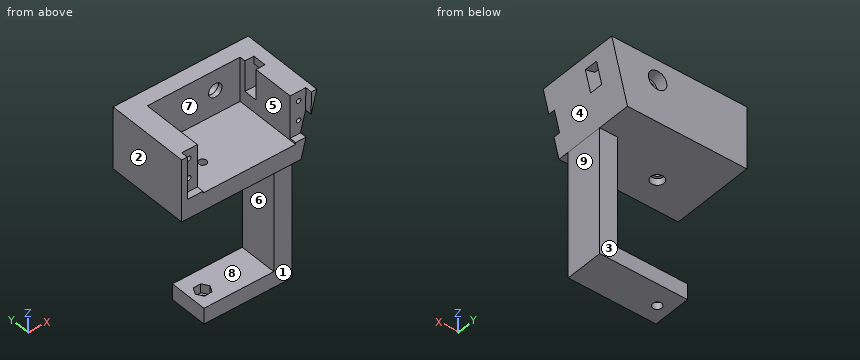
Autodesk Inventor part; units mm, degrees
ref_plane "Work Plane4" through (-33.8514, -22.438, 35.052) normal (0, 0, 1) x (0, 1, 0)
ref_plane "YZ Plane" through (0, 0, 0) normal (1, 0, 0) x (0, 1, 0)
ref_plane "XZ Plane" through (0, 0, 0) normal (0, 1, 0) x (-1, 0, 0)
sketch "Sketch1" plane through (0, 0, 0) normal (0, 0, 1) x (1, 0, 0)
  line L0 (-33.8514, 24.552) -> (33.4586, 24.552)
  line L1 (33.4586, 24.552) -> (33.4586, -22.438)
  line L2 (33.4586, -22.438) -> (-33.8514, -22.438)
  line L3 (-33.8514, -22.438) -> (-33.8514, 24.552)
  line L4 (33.4586, -22.438) -> (33.4586, -16.088)
  line L5 (33.4586, -16.088) -> (23.2986, -16.088)
  line L6 (23.2986, -16.088) -> (23.2986, 5.502)
  line L7 (23.2986, 5.502) -> (33.4586, 5.502)
  point P0 (0, 0)
  dimension "d0" = 67.31
  dimension "d1" = 46.99
  dimension "d10" = 6.35
  dimension "d11" = 10.16
  dimension "d12" = 21.59
ref_plane "Work Plane3" through (-33.8514, -22.438, 0) normal (0, 0, 1) x (0, 1, 0)
ref_plane "Work Plane4" through (-33.8514, -22.438, 35.052) normal (0, 0, 1) x (0, 1, 0)
sketch "Sketch3" plane through (-33.8514, -22.438, 35.052) normal (0, 0, 1) x (0, 1, 0)
  line L0 (0, 0) -> (46.99, 0)
  line L1 (46.99, 0) -> (46.99, -76.2)
  line L2 (46.99, -76.2) -> (0, -76.2)
  line L3 (0, -76.2) -> (0, 0)
  point P0 (22.438, -33.8514)
  dimension "d4" = 46.99
  dimension "d5" = 76.2
loft "Loft1" add profiles "Sketch3", "Sketch1"
sketch "Sketch5" plane through (33.4586, -22.438, 0) normal (0, 0, -1) x (-1, 0, 0)
  line L0 (67.31, 0) -> (67.31, 46.99)
  line L1 (-8.89, 0) -> (67.31, 0)
  circle A0 centre (42.037, 16.383) radius 3.683
  circle A1 centre (42.037, 16.383) radius 2.159
  point P0 (33.4586, 22.438)
  dimension "d17" = 7.366
  dimension "d20" = 4.318
extrude "Extrusion1" add sketch "Sketch1" against normal blind 71.12 contours L1 L5 L6 L7
extrude "Extrusion4" cut sketch "Sketch5" along normal through all both and the other way through all contours A1
extrude "Extrusion5" cut sketch "Sketch5" against normal blind 3.81 contours A0 | A1
sketch "Sketch7" plane through (23.2986, -16.088, 0) normal (-1, 0, 0) x (0, 0, 1)
  point P0 (0, 16.088)
sketch "Sketch8" plane through (23.2986, -16.088, 0) normal (-1, 0, 0) x (0, 0, 1)
  line L0 (0, 0) -> (-71.12, 0)
  line L1 (0, 21.59) -> (-71.12, 21.59)
  line L2 (-71.12, 0) -> (-62.23, 0)
  line L3 (-62.23, 0) -> (-62.23, 21.59)
  line L4 (-62.23, 21.59) -> (-71.12, 21.59)
  line L5 (-71.12, 21.59) -> (-71.12, 0)
  point P0 (0, 16.088)
  dimension "d27" = 8.89
extrude "Extrusion6" add sketch "Sketch8" along normal blind 39.37
sketch "Sketch9" plane through (0, 0, -71.12) normal (0, 0, -1) x (-1, 0, 0)
  line L0 (16.0714, 5.502) -> (16.0714, -16.088)
  line L1 (-33.4586, -16.088) -> (16.0714, -16.088)
  circle A0 centre (8.5784, -6.055) radius 2.54
  point P0 (0, 0)
  dimension "d34" = 5.08
extrude "Extrusion7" cut sketch "Sketch9" against normal blind 39.37
sketch "Sketch10" plane through (-33.8514, -22.438, 35.052) normal (0, -1, 0) x (1, 0, 0)
  line L0 (67.31, -35.052) -> (67.31, -106.172)
  line L1 (67.31, -35.052) -> (70.1199, -23.9728)
  line L2 (76.2, 0) -> (67.31, -35.052)
  line L3 (70.1199, -23.9728) -> (64.2779, -23.9728)
  line L4 (64.2779, -23.9728) -> (64.2779, -24.9888)
  line L5 (64.2779, -24.9888) -> (11.9539, -24.9888)
  line L6 (11.9539, -24.9888) -> (11.9539, -23.9728)
  line L7 (11.9539, -23.9728) -> (3.1655, -23.9728)
  line L8 (3.1655, -23.9728) -> (3.1655, 0)
  line L9 (0, 0) -> (76.2, 0)
  line L10 (76.2, 0) -> (73.0154, -12.5564)
  line L11 (76.2, 0) -> (73.152, 0)
  line L12 (73.152, 0) -> (73.0154, -12.5564)
  line L13 (73.0154, -12.5564) -> (70.1199, -23.9728)
  line L14 (73.152, 0) -> (3.1655, 0)
  line L15 (11.9539, -23.9728) -> (11.9539, 0)
  line L16 (64.2779, -23.9728) -> (64.2779, 0)
  line L17 (11.9539, 0) -> (7.1279, 0)
  circle A0 centre (7.1279, -5.334) radius 1.27
  line L18 (11.9539, -23.9728) -> (7.1279, -23.9728)
  circle A1 centre (7.1279, -16.3528) radius 1.27
  line L19 (73.152, 0) -> (68.326, 0)
  line L20 (64.2779, 0) -> (69.1039, 0)
  circle A2 centre (69.1039, -5.334) radius 1.27
  line L21 (64.2779, -23.9728) -> (69.1039, -23.9728)
  circle A3 centre (69.1039, -16.3528) radius 1.27
  point P0 (33.8514, -35.052)
  point P1 (64.2779, 0)
  point P2 (11.9539, 0)
  dimension "d37" = 11.43
  dimension "d38" = 5.842
  dimension "d39" = 1.016
  dimension "d40" = 52.324
  dimension "d41" = 8.7884
  dimension "d42" = 12.954
  dimension "d43" = 3.048
  dimension "d48" = 4.826
  dimension "d50" = 2.54
  dimension "d52" = 2.54
  dimension "d56" = 4.826
  dimension "d58" = 2.54
  dimension "d59" = 4.826
  dimension "d61" = 2.54
extrude "Extrusion8" cut sketch "Sketch10" against normal blind 38.1 contours L4 L5 L6 L15 L9 L16
extrude "Extrusion9" cut sketch "Sketch10" against normal blind 3.81 contours L2 L3 L16 L9 L12 | L15 L7 L8 L9 | A0 | A1 | A2 | A3
sketch "Sketch15" plane through (-33.8514, -18.628, 35.052) normal (0, -1, 0) x (1, 0, 0)
  line L0 (11.9539, -24.9888) -> (11.9539, 0)
  line L1 (11.9539, -23.9729) -> (11.9539, -16.3529)
  line L2 (11.9539, -16.3529) -> (7.1279, -16.3529)
  circle A0 centre (7.1279, -16.3529) radius 1.27
  line L3 (11.9539, 0) -> (64.2779, 0)
  line L4 (11.9539, 0) -> (7.1279, 0)
  line L5 (3.1655, 0) -> (11.9539, 0)
  circle A1 centre (7.1279, -5.334) radius 1.27
  point P0 (33.8514, -35.052)
  dimension "d64" = 7.62
  dimension "d65" = 4.826
  dimension "d66" = 2.54
  dimension "d70" = 2.54
extrude "Extrusion11" cut sketch "Sketch15" against normal blind 10.16 contours A0
sketch "Sketch14" plane through (-33.8514, -18.628, 35.052) normal (0, -1, 0) x (1, 0, 0)
  point P0 (33.8514, -35.052)
extrude "Extrusion12" cut sketch "Sketch15" against normal blind 10.16 contours A1
sketch "Sketch16" plane through (-33.8514, -18.628, 35.052) normal (0, -1, 0) x (1, 0, 0)
  line L0 (11.9539, 0) -> (64.2779, 0)
  line L1 (64.2779, 0) -> (69.1039, 0)
  line L2 (0, 0) -> (76.2, 0)
  circle A0 centre (69.1039, -5.334) radius 1.27
  line L3 (64.2779, -23.9728) -> (64.2779, -24.9888)
  line L4 (64.2779, -23.9728) -> (69.1039, -23.9728)
  line L5 (70.1199, -23.9728) -> (64.2779, -23.9728)
  circle A1 centre (69.1039, -16.3528) radius 1.27
  point P0 (33.8514, -35.052)
  dimension "d73" = 4.826
  dimension "d75" = 2.54
  dimension "d76" = 4.826
  dimension "d78" = 2.54
extrude "Extrusion13" cut sketch "Sketch16" against normal blind 10.16
sketch "Sketch17" plane through (-33.8514, 15.662, 35.052) normal (0, -1, 0) x (1, 0, 0)
  line L0 (64.2779, -23.9728) -> (64.2779, 0)
  line L1 (64.2779, 0) -> (50.3079, 0)
  line L2 (11.9539, 0) -> (64.2779, 0)
  circle A0 centre (50.3079, -11.43) radius 3.81
  point P0 (33.8514, -35.052)
  dimension "d81" = 13.97
  dimension "d83" = 7.62
extrude "Extrusion14" cut sketch "Sketch17" against normal through all
sketch "Sketch18" plane through (-33.8514, 24.552, 35.052) normal (0, 1, 0) x (1, 0, 0)
  circle A0 centre (50.3079, 11.43) radius 3.81
  circle A1 centre (50.3079, 11.43) radius 5.207
  point P0 (33.8514, 35.052)
  dimension "d86" = 10.414
extrude "Extrusion15" cut sketch "Sketch18" against normal blind 6.35 contours A0 | A1
sketch "Sketch19" plane through (30.4266, -22.438, 10.0632) normal (-1, 0, 0) x (0, 0, 1)
  line L0 (24.9888, 38.1) -> (0, 38.1)
  line L1 (24.9888, 38.1) -> (24.9888, 3.81)
  line L2 (24.9888, 34.798) -> (7.7168, 34.798)
  line L3 (7.7168, 34.798) -> (7.7168, 27.178)
  line L4 (7.7168, 27.178) -> (24.9888, 27.178)
  point P0 (-10.0632, 22.438)
  dimension "d89" = 3.302
  dimension "d90" = 17.272
  dimension "d91" = 7.62
extrude "Extrusion16" cut sketch "Sketch19" against normal blind 5.08
sketch "Sketch20" plane through (42.3486, -22.438, 35.052) normal (0.9693105, 0, -0.2458396) x (-0.2458396, 0, -0.9693105)
  line L0 (0, 46.99) -> (36.1618, 46.99)
  line L1 (0, 46.99) -> (0, 34.798)
  line L2 (0, 46.99) -> (0, 0)
  line L3 (0, 34.798) -> (5.842, 34.798) construction
  line L4 (5.842, 34.798) -> (5.842, 27.178)
  line L5 (5.842, 27.178) -> (17.526, 27.178)
  line L6 (17.526, 27.178) -> (17.526, 34.798)
  line L7 (17.526, 34.798) -> (5.842, 34.798)
  point P0 (44.3872, 22.438)
  dimension "d94" = 12.192
  dimension "d98" = 11.684
extrude "Extrusion17" cut sketch "Sketch20" against normal blind 11.938
sketch "Sketch21" plane through (35.5066, -22.438, 10.0632) normal (-1, 0, 0) x (0, 0, 1)
  line L0 (7.7168, 27.178) -> (7.7168, 34.798)
  line L1 (7.7168, 34.798) -> (8.6432, 34.798)
  line L2 (7.7168, 34.798) -> (8.6432, 34.798)
  line L3 (8.6432, 27.178) -> (8.6432, 34.798)
  line L4 (8.6432, 34.798) -> (8.6432, 27.178)
  line L5 (24.9888, 27.178) -> (7.7168, 27.178)
  line L6 (8.6432, 27.178) -> (7.7168, 27.178)
  line L7 (7.7168, 27.178) -> (7.7168, 34.798)
  point P0 (-10.0632, 22.438)
extrude "Extrusion18" cut sketch "Sketch21" against normal blind 11.938
sketch "Sketch22" plane through (23.2986, -16.088, -62.23) normal (0, 0, 1) x (1, 0, 0)
  circle A0 centre (-31.877, 10.033) radius 2.54
  line L0 (-29.5969, 6.3661) -> (-33.9126, 6.2249)
  line L1 (-33.9126, 6.2249) -> (-36.1927, 9.8919)
  line L2 (-36.1927, 9.8919) -> (-34.1571, 13.6999)
  line L3 (-34.1571, 13.6999) -> (-29.8414, 13.8411)
  line L4 (-29.8414, 13.8411) -> (-27.5613, 10.1741)
  line L5 (-27.5613, 10.1741) -> (-29.5969, 6.3661)
  point P0 (-23.2986, 16.088)
extrude "Extrusion20" cut sketch "Sketch22" against normal blind 5.08 contours A0 | L0 L1 L2 L3 L4 L5
Work out the finished part from the listing and answer in its coordinate system (mm). Face numbers are marked on the shaded views. A direction names the side the tool comes from. Round coordinates to 2 decimals unless told otherwise and drop trailing zeros. Order: outer loops, then holes, each group sorted by start corner. A loop starts at its lowest first (then second) coordinate and runs counter-clockwise, first axis right, second up. Notation, with made-up numbers: M 47.25,-26 L 82.25,-26 A18 cw 82.25,-2 Z; hole C -18,49 d9. An arc over 180 degrees is marked long. One line per item, written item: value.
Q1. Find section B-B on z = -15.5. Write down the section's boundary in (x, y), then the cut area to 3 significant figures.
Derived:
outline: M 23.3,-16.09 L 33.46,-16.09 L 33.46,5.5 L 23.3,5.5 Z
area: 219 mm²
Q2. For the marked faces 1, 2, 3, 4 and 5, determine the directions among +Z, -Z, +X, -X, +Y, -Y from which every point of the face is accessible in a straight line to the end or side of a thin tool.
Derived:
face 1: -Z, +X, -X, -Y
face 2: +Z, -Z, -X, +Y, -Y
face 3: -Z, +X, -X, +Y
face 4: -Z, +X, +Y, -Y
face 5: +Z, -Y
Q3. Find section C-C on x = 14. Give the number of separate pieces and of enclosed holes in the cut face, then the cut area to 3 significant figures.
Derived:
separate pieces: 3
enclosed holes: 0
area: 814 mm²
Q4. Determine the mould class of the marked faces 6, 7, 8 and 9 for opening direction X: released by +X, released by -X, zero draft, split by the parting line, or undercut.
Derived:
face 6: released by -X
face 7: undercut
face 8: zero draft
face 9: released by +X
Q5. Flat-ended cylindrical pins translate along their axes: pin 1 (6 mm diameter, centred on x = 34, y = -17, fed in from -Z); pin 2 (2 mm diameter, centred on x = 31, z = -16.5, fed in from -Y); pin 3 (9 mm diameter, centred on x = 16.46, z = 23.62, fed in from +Y); pin 4 (3 mm diameter, centred on x = 35, z = 23.5, fed in from -Y). Find the tip coordinate at first contact, or state that the pin passes through.
Derived:
pin 1: z = -71.12
pin 2: y = -16.09
pin 3: y = 18.2
pin 4: y = -18.63
Q6. Straight lines are drawn through the part: line 1 (Z direction, x = 9, y = -10.5); line 2 (X direction, y = -17.5, z = 29); line 3 (X direction, y = -2, z = -20.5). For each, find the intervals that lie inside material, in ascending order.
Derived:
line 1: -71.12 to -62.23, 0 to 10.06
line 2: -33.85 to -27.77, -25.68 to -21.9, 30.43 to 34.2, 36.3 to 40.81
line 3: 23.3 to 33.46
Q7. Find section A-A on y = -11. Write down the section's boundary in (x, z), then the cut area to 3 significant figures.
Derived:
outline: M -33.85,0 L 23.3,0 L 23.3,-62.23 L -16.07,-62.23 L -16.07,-71.12 L 33.46,-71.12 L 33.46,0 L 42.35,35.05 L 30.43,35.05 L 30.43,10.06 L -21.9,10.06 L -21.9,35.05 L -33.85,35.05 Z; hole C -26.72,18.7 d2.54; hole C -26.72,29.72 d2.54; hole C 35.25,18.7 d2.54; hole C 35.25,29.72 d2.54
area: 2,260 mm²
